```python
from build123d import *

# Parameters (mm, degrees)
SKETCH_1_R               = 1.5
EXTRUDE_1_DEPTH          = 10
CUT_EXTRUDE_1_DEPTH      = 3
CUT_EXTRUDE_1_DEPTH_BACK = 3
SKETCH_2_R               = 2.7


with BuildPart() as part:
    # 草图1 → 凸台-拉伸1 (new body)
    with BuildSketch(Plane(origin=(0, 0, 0), x_dir=(1, 0, 0), z_dir=(0, 1, 0))):
        with BuildLine():
            Line((-1.4, -2.308679276), (-1.4, -13.691320724))
            ThreePointArc((-1.4, -13.691320724), (0, -18.7), (1.4, -13.691320724))
            Line((1.4, -13.691320724), (1.4, -2.308679276))
            ThreePointArc((1.4, -2.308679276), (0, 2.7), (-1.4, -2.308679276))
        make_face()
        with Locations(Location((0, 0, 0), (0, 0, 270))):
            Circle(SKETCH_1_R, mode=Mode.SUBTRACT)
        with Locations(Location((0, -16, 0), (0, 0, 270))):
            Circle(SKETCH_1_R, mode=Mode.SUBTRACT)
    extrude(amount=EXTRUDE_1_DEPTH)

    # 草图2 → 切除-拉伸1 (cut, two sides: drawn at the far end of the back side and taken through both)
    with BuildSketch(Plane(origin=(0, 5, 0), x_dir=(-1, 0, 0), z_dir=(0, -1, 0)).offset(-CUT_EXTRUDE_1_DEPTH_BACK)):
        with BuildLine():
            Line((-1.4, -2.308679276), (-1.4, -3))
            Line((-1.4, -3), (1.4, -3))
            Line((1.4, -3), (1.4, -2.308679276))
            ThreePointArc((1.4, -2.308679276), (0, -2.7), (-1.4, -2.308679276))
        make_face()
        Circle(SKETCH_2_R)
    extrude(amount=CUT_EXTRUDE_1_DEPTH + CUT_EXTRUDE_1_DEPTH_BACK, mode=Mode.SUBTRACT)


solid = part.part
```
Verification items for the finished model (mm, model axes). A direction names the side the tool comes from. Give positions to 0.01 mm unless a question says otherwise; leave off trailing zeros. Order: outer loops, then holes, each group sorted by start corner. A loop starts at its lowest first (then second) coordinate and runs counter-clockwise, first axis right, second up. Notation, with made-up numbers: (64, 66.5) -> (93, 66.5) arc R21 ccw to (93, 105.5) -> close; hole circle Ø6 at (87, 89). An arc over 180 degrees is marked (long way). One line per item, written item: value.
(1) Sectioned sample at B-B on x = 0. Record the cut outline in (y, z).
Final values:
outline: (0, -2.7) -> (2, -2.7) -> (2, -1.5) -> (0, -1.5) -> close; (0, 1.5) -> (2, 1.5) -> (2, 3) -> (8, 3) -> (8, 1.5) -> (10, 1.5) -> (10, 14.5) -> (0, 14.5) -> close; (0, 17.5) -> (10, 17.5) -> (10, 18.7) -> (0, 18.7) -> close; (8, -2.7) -> (10, -2.7) -> (10, -1.5) -> (8, -1.5) -> close
(2) Gauge pin test, flat ends, axial feed: pin 1 (3 mm diameter, centred on x = 0, y = 4.5, fed in from -Z); pin 2 (3 mm diameter, centred on y = 4, z = 5.5, fed in from +X). Record the tip position at first contact, or that the pin passes through.
Final values:
pin 1: z = 3
pin 2: x = 1.4
(3) Tool access check on faces 1 (the face through (-1.4, 5, 8)), 2 (the face through (-1.2, 8, -1.2)), 3 (the face through (1.4, 5, 8)). Record the directions out of +Z, -Z, +X, -X, +Y, -Y that give a thin tool (end or side, any length) a straight path to the whole face; none if there is none.
Final values:
face 1: -X, +Y, -Y
face 2: -Z, +X, -X
face 3: +X, +Y, -Y
(4) Sectioned sample at D-D on y = 9.25. Record the cut outline in (x, z).
Final values:
outline: (-1.4, 2.31) arc R2.7 ccw (long way) to (1.4, 2.31) -> (1.4, 13.69) arc R2.7 ccw (long way) to (-1.4, 13.69) -> close; hole circle Ø3 at (0, 0); hole circle Ø3 at (0, 16)
(5) Scan lines: line 1 along X through (y, z) = (2.75, 16); line 2 along Y through (x, z) = (1.15, -1); line 3 along X through (y, z) = (4.75, 4.25). Record each from-to range of solid material in increasing order. Write a range as [from, to].
Final values:
line 1: [-2.7, -1.5], [1.5, 2.7]
line 2: [0, 2], [8, 10]
line 3: [-1.4, 1.4]
(6) Draft check along Z on faces 4 (the face through (0.1, 9, -2.7)), 5 (the face through (0, 5, 3)), 6 (the face through (0, 10, 8)). Enter one of: pulls with the +Z half, pulls with the -Z half, needs draft (parallel to the pull), parting line crosses it, or undercut.
Final values:
face 4: undercut
face 5: pulls with the -Z half
face 6: needs draft
(7) Sectioned sample at A-A on z = 0. Record the cut outline in (x, y).
Final values:
outline: (-2.7, 0) -> (-1.5, 0) -> (-1.5, 2) -> (-2.7, 2) -> close; (-2.7, 8) -> (-1.5, 8) -> (-1.5, 10) -> (-2.7, 10) -> close; (1.5, 0) -> (2.7, 0) -> (2.7, 2) -> (1.5, 2) -> close; (1.5, 8) -> (2.7, 8) -> (2.7, 10) -> (1.5, 10) -> close
(8) Sectioned sample at C-C on z = 16. Record the cut outline in (x, y).
Final values:
outline: (-2.7, 0) -> (-1.5, 0) -> (-1.5, 10) -> (-2.7, 10) -> close; (1.5, 0) -> (2.7, 0) -> (2.7, 10) -> (1.5, 10) -> close
